Work out the finished part from the listing and answer in its coordinate system (mm). Round coordinates to 2 decimals unless told otherwise and drop trailing zeros. Write each loop counter-clockwise with the first axis right and the second up, starting at its lowest first coordinate (ties: lowest second). Pieces come first, ordered by that corner, then holes. Notation, with made-up numbers: (-31.5, 2) -> (-22.5, 2) arc R31 cw to (-22.5, 29) -> close; hole circle Ø7 at (86, -15). An arc over 180 degrees is marked (long way). One line per item, written item: value.
```python
from build123d import *

# Parameters (mm, degrees)
SKETCH1_W           = 900
SKETCH1_H           = 600
BOSS_EXTRUDE1_DEPTH = 30
SKETCH2_W           = 100
SKETCH2_H           = 100
CUT_EXTRUDE1_DEPTH  = 623.016629111
SKETCH4_R           = 10
SKETCH4_W           = 20
SKETCH4_H           = 20
CUT_EXTRUDE2_DEPTH  = 176
SKETCH5_W           = 415
SKETCH5_H           = 70
CUT_EXTRUDE3_DEPTH  = 110


with BuildPart() as part:
    # Sketch1 → Boss-Extrude1 (new body)
    with BuildSketch(Plane(origin=(0, 0, 0), x_dir=(1, 0, 0), z_dir=(0, 1, 0))):
        with Locations((48.214762953, -71.196358908)):
            Rectangle(SKETCH1_W, SKETCH1_H)
    extrude(amount=BOSS_EXTRUDE1_DEPTH)

    # Sketch2 → Cut-Extrude1 (cut, through all)
    with BuildSketch(Plane(origin=(0, 30, 0), x_dir=(1, 0, 0), z_dir=(0, 1, 0))):
        with Locations((-351.785237047, 178.803641092)):
            Rectangle(SKETCH2_W, SKETCH2_H)
        with Locations((-351.785237047, -321.196358908)):
            Rectangle(SKETCH2_W, SKETCH2_H)
        with Locations((448.214762953, -321.196358908)):
            Rectangle(SKETCH2_W, SKETCH2_H)
        with Locations((448.214762953, 178.803641092)):
            Rectangle(SKETCH2_W, SKETCH2_H)
    extrude(amount=-CUT_EXTRUDE1_DEPTH, mode=Mode.SUBTRACT)

    # Sketch4 → Cut-Extrude2 (cut)
    with BuildSketch(Plane(origin=(0, 30, 0), x_dir=(1, 0, 0), z_dir=(0, 1, 0))):
        with Locations(Location((-342.785237047, -71.196358908, 0), (0, 0, 270))):
            Circle(SKETCH4_R)
        with Locations((-86.285237047, -71.196358908)):
            Rectangle(SKETCH4_W, SKETCH4_H)
    extrude(amount=-CUT_EXTRUDE2_DEPTH, mode=Mode.SUBTRACT)

    # Sketch5 → Cut-Extrude3 (cut)
    with BuildSketch(Plane(origin=(0, 30, 0), x_dir=(1, 0, 0), z_dir=(0, 1, 0))):
        with Locations((235.714762953, -66.196358908)):
            Rectangle(SKETCH5_W, SKETCH5_H)
    extrude(amount=-CUT_EXTRUDE3_DEPTH, mode=Mode.SUBTRACT)


solid = part.part
```
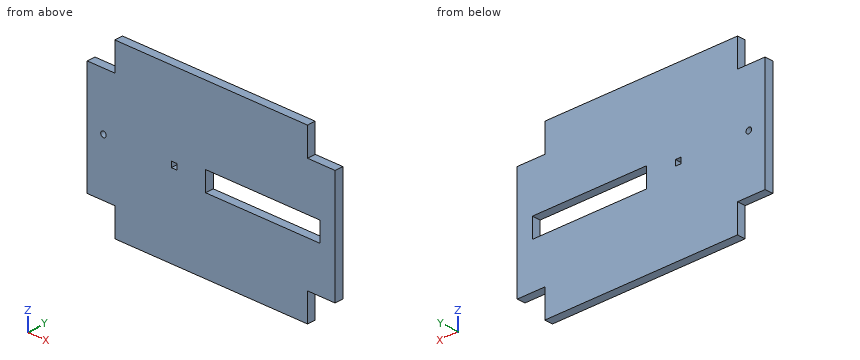
(1) Find section A-A on x = 115.5. Give the vertices of the cut face in (y, z).
Reported:
outline: (0, -228.8) -> (30, -228.8) -> (30, 31.2) -> (0, 31.2) -> close; (0, 101.2) -> (30, 101.2) -> (30, 371.2) -> (0, 371.2) -> close
(2) Flat-ended cylindrical pins translate along their axes: pin 1 Ø15 at (x, y) = (463.5, 16.5) entering from +Z; pin 2 Ø9 at (x, y) = (-363, 9) entering from -Z; pin 3 Ø4 at (y, z) = (25, 286.5) entering from -X. Find the tip coordinate at first contact, or state that the pin passes through.
Reported:
pin 1: stops at z = 271.2
pin 2: stops at z = -128.8
pin 3: stops at x = -301.79
(3) Consider probe 1 along Z at (x, y) = (57, 9.75); probe 2 along X at (y, z) = (26.5, 92.5); probe 3 along X at (y, z) = (3.75, -132.5). Determine where each line is inside the solid, lowest interval first.
Reported:
probe 1: z = -228.8 to 31.2, 101.2 to 371.2
probe 2: x = -401.79 to 28.21, 443.21 to 498.21
probe 3: x = -301.79 to 398.21
(4) Find section C-C on z = -170. Give the vertices of the cut face in (x, y), plus the area to 3 significant figures.
Reported:
outline: (-301.79, 0) -> (398.21, 0) -> (398.21, 30) -> (-301.79, 30) -> close
area: 21,000 mm2
(5) Find section B-B on y = 5.5. Give the vertices of the cut face in (x, z).
Reported:
outline: (-401.79, -128.8) -> (-301.79, -128.8) -> (-301.79, -228.8) -> (398.21, -228.8) -> (398.21, -128.8) -> (498.21, -128.8) -> (498.21, 271.2) -> (398.21, 271.2) -> (398.21, 371.2) -> (-301.79, 371.2) -> (-301.79, 271.2) -> (-401.79, 271.2) -> close; hole circle Ø20 at (-342.79, 71.2); hole (-96.29, 61.2) -> (-76.29, 61.2) -> (-76.29, 81.2) -> (-96.29, 81.2) -> close; hole (28.21, 31.2) -> (443.21, 31.2) -> (443.21, 101.2) -> (28.21, 101.2) -> close
